Study the drawing (mm; zero at the part's minimum x, y, z) and answer. A direction names the side the tool comes from. Round coordinates to 2 decimals unless told otherwise and drop trailing zeros. Write each loop counter-clockwise with the first axis right and the second up, starting at its lowest first coordinate (ties: lowest second). Pieces come first, ordered by that corner, then holes.
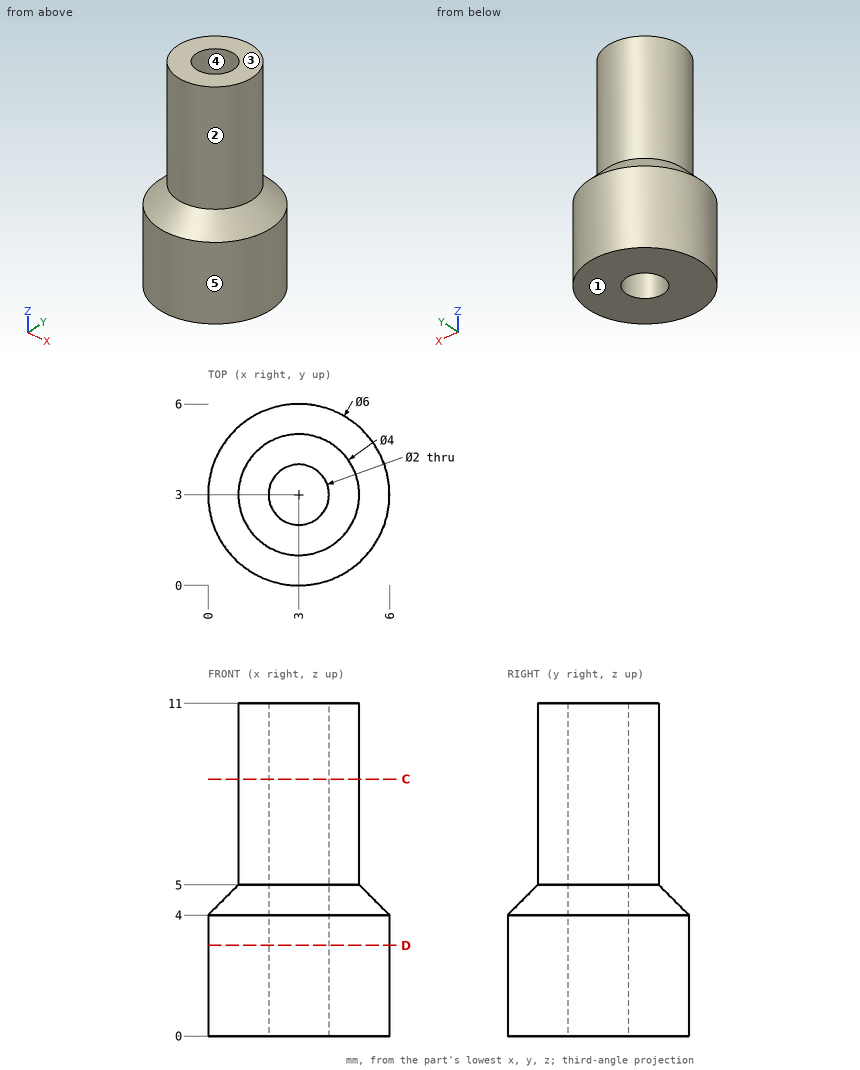
1. Given pin 1 (3 mm diameter, centred on y = 2, z = 7, fed in from +X); pin 2 (2 mm diameter, centred on y = 4.5, z = 8.5, fed in from +X), each flat-ended and moving along its own axis, determine where each tip first touches the part or whether it passes through.
Geometry says:
pin 1: stops at x = 5
pin 2: stops at x = 4.94
2. Straight lines are drawn through the part: line 1 along Y through (x, z) = (3, 5.5); line 2 along X through (y, z) = (3.55, 7.75) (1 decimal); line 3 along Y through (x, z) = (2.75, 4.25). For each, find the intervals that lie inside material, in ascending order.
Geometry says:
line 1: y = 1 to 2, 4 to 5
line 2: x = 1.1 to 2.2, 3.8 to 4.9
line 3: y = 0.26 to 2.03, 3.97 to 5.74
3. Section D-D on z = 3 is taken. Determine the outline of the cut face in (x, y).
Geometry says:
outline: circle Ø6 at (3, 3); hole circle Ø2 at (3, 3)
4. Section C-C on z = 8.5 is taken. Determine the outline of the cut face in (x, y).
Geometry says:
outline: circle Ø4 at (3, 3); hole circle Ø2 at (3, 3)
5. For a pull along Y with two mould halves and no side action, classify the marked faces 3, 4 and 5 as released by +Y, released by -Y, zero draft, split by the parting line, or undercut.
Geometry says:
face 3: zero draft
face 4: undercut
face 5: split by the parting line
6. A tool of negligible diameter and unlimited length cuts with its end or side. For the marked faces 1 and 2, from which of +Z, -Z, +X, -X, +Y, -Y can it reach the whole face along a straight path? Write none if from no direction.
Geometry says:
face 1: -Z, +X, -X, +Y, -Y
face 2: +Z
